Autodesk Inventor part; units mm, degrees
ref_plane "YZ Plane" through (0, 0, 0) normal (1, 0, 0) x (0, 1, 0)
ref_plane "XZ Plane" through (0, 0, 0) normal (0, 1, 0) x (-1, 0, 0)
ref_plane "XY Plane" through (0, 0, 0) normal (0, 0, 1) x (1, 0, 0)
sketch "Sketch1" plane through (0, 0, 0) normal (0, 0, 1) x (1, 0, 0)
  line L0 (-25, -20) -> (25, -20)
  line L1 (25, -20) -> (25, 20)
  line L2 (25, 20) -> (-25, 20)
  line L3 (-25, 20) -> (-25, -20)
  point P0 (0, 0)
  dimension "d0" = 50
  dimension "d1" = 40
extrude "Extrusion1" add sketch "Sketch1" along normal blind 6.5
sketch "Sketch2" plane through (0, 0, 6.5) normal (0, 0, 1) x (1, 0, 0)
  circle A0 centre (-15, 0) radius 3.25
  point P0 (0, 0)
  dimension "d4" = 6.5
hole "Hole1" at (-15, 0, 6.5) direction (0, 0, -1) diameter 6.5 end through all
sketch "Sketch3" plane through (0, 0, 6.5) normal (0, 0, 1) x (1, 0, 0)
  circle A0 centre (15, 0) radius 3.25
  point P0 (0, 0)
  dimension "d12" = 6.5
hole "Hole2" at (15, 0, 6.5) direction (0, 0, -1) diameter 6.5 end through all
properties part number "Bed Plate"
Build history of the part. All positions in model axes, mm. Round coordinates to 2 decimals unless told otherwise and drop trailing zeros. Write each loop counter-clockwise with the first axis right and the second up, starting at its lowest first coordinate (ties: lowest second). Pieces come first, ordered by that corner, then holes. Notation, with made-up numbers: M 40.5,33.5 L 71.5,33.5 A28 cw 71.5,56.5 Z; hole C -1,52.5 d4. An arc over 180 degrees is marked long. Answer as a JSON object with one key per item and string values. Group by question number.
(1) Cut at D-D (x = -13). Give the cut face in (y, z).
(2) Drill centre lines: L1, parallel to X at y = 0, z = 3.75; L2, parallel to Y at x = -15, z = 3.25; L3, parallel to Y at x = 12.5, z = 2.25. Where is each one in solid material? Low to high.
(3) Cut at A-A (x = 15). Give the cut face in (y, z), and give its area (3 significant figures).
(4) Mould opens along Y. For faces 1 (the flat face through (25, 0, 3)), 2 (the flat face through (0, -20, 3)), 3 (the cylindrical face through (-18.222, 0.423, 3.204)), 4 (the flat face through (0, 20, 3)) say: pulls with the +Y half, pulls with the -Y half, needs draft (parallel to the pull), parting line crosses it, or undercut.
(5) Cut at B-B (y = 0). Give the cut face in (x, z), and give its area (4 significant figures).
(6) Cut at C-C (z = 1.25). Give the cut face in (x, y).
(7) Flat gauge pin, fed straight in: pin 1 (6 mm diameter, centred on x = -15, y = 0, fed in from -Z). Where does the tip first touch, or does it go through?
Responses:
{
 "1": {"outline": "M -20,0 L -2.56,0 L -2.56,6.5 L -20,6.5 Z; M 2.56,0 L 20,0 L 20,6.5 L 2.56,6.5 Z"},
 "2": {"L1": "x = -25 to -18.25, -11.75 to 11.75, 18.25 to 25", "L2": "y = -20 to -3.25, 3.25 to 20", "L3": "y = -20 to -2.08, 2.08 to 20"},
 "3": {"outline": "M -20,0 L -3.25,0 L -3.25,6.5 L -20,6.5 Z; M 3.25,0 L 20,0 L 20,6.5 L 3.25,6.5 Z", "area": "218 mm2"},
 "4": {"face 1": "needs draft", "face 2": "pulls with the -Y half", "face 3": "undercut", "face 4": "pulls with the +Y half"},
 "5": {"outline": "M -25,0 L -18.25,0 L -18.25,6.5 L -25,6.5 Z; M -11.75,0 L 11.75,0 L 11.75,6.5 L -11.75,6.5 Z; M 18.25,0 L 25,0 L 25,6.5 L 18.25,6.5 Z", "area": "240.5 mm2"},
 "6": {"outline": "M -25,-20 L 25,-20 L 25,20 L -25,20 Z; hole C -15,0 d6.5; hole C 15,0 d6.5"},
 "7": {"pin 1": "passes through"}
}
